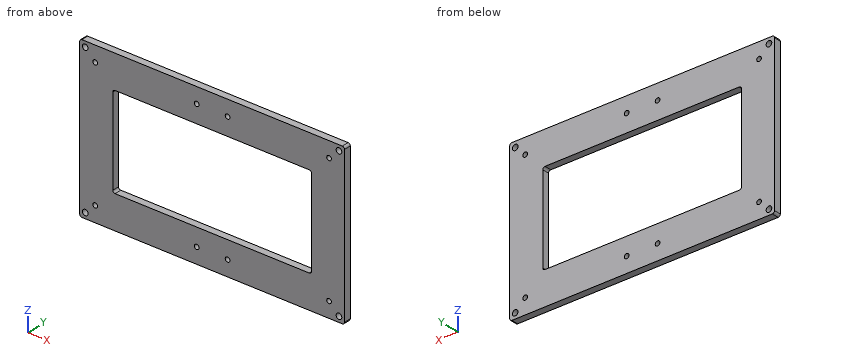
Autodesk Inventor part; units mm, degrees
ref_plane "YZ Plane" through (0, 0, 0) normal (1, 0, 0) x (0, 1, 0)
ref_plane "XZ Plane" through (0, 0, 0) normal (0, 1, 0) x (-1, 0, 0)
ref_plane "XY Plane" through (0, 0, 0) normal (0, 0, 1) x (1, 0, 0)
sketch "Sketch1" plane through (0, 0, 0) normal (0, 1, 0) x (-1, 0, 0)
  line L0 (-120, 71.5) -> (120, 71.5)
  line L1 (120, 71.5) -> (120, 41.5)
  line L2 (120, 41.5) -> (-120, 41.5)
  line L3 (-120, 41.5) -> (-120, 71.5)
  line L4 (-120, -41.5) -> (120, -41.5)
  line L5 (120, -41.5) -> (120, -71.5)
  line L6 (120, -71.5) -> (-120, -71.5)
  line L7 (-120, -71.5) -> (-120, -41.5)
  line L8 (168, 0) -> (-168, 0)
  line L9 (0, -100.1) -> (0, 100.1)
  line L10 (120, 41.5) -> (-120, 41.5)
  line L11 (-120, 41.5) -> (-120, -41.5)
  line L12 (-120, -41.5) -> (120, -41.5)
  line L13 (120, -41.5) -> (120, 41.5)
  line L14 (90, 41.5) -> (-90, 41.5)
  line L15 (-90, 41.5) -> (-90, -41.5)
  line L16 (-90, -41.5) -> (90, -41.5)
  line L17 (90, -41.5) -> (90, 41.5)
  line L18 (-115, 66.5) -> (115, 66.5) construction
  line L19 (115, 66.5) -> (115, -66.5) construction
  line L20 (115, -66.5) -> (-115, -66.5) construction
  line L21 (-115, -66.5) -> (-115, 66.5) construction
  point P0 (0, 0)
  point P1 (0, 41.5)
  dimension "d0" = 240
  dimension "d2" = 30
  dimension "d4" = 143
  dimension "d55" = 30
  dimension "d56" = 5
  dimension "d57" = 5
extrude "Extrusion1" add sketch "Sketch1" along normal blind 6.35 contours L0 L9 L2 L3 | L0 L1 L2 L9 | L2 L15 L8 L11 | L8 L15 L4 L11 | L13 L8 L17 L2 | L4 L9 L6 L7 | L13 L4 L17 L8 | L4 L5 L6 L9
sketch "Sketch2" plane through (0, 6.35, 0) normal (0, 1, 0) x (1, 0, 0)
  line L0 (-110, -61.5) -> (-10, -61.5)
  line L1 (-10, -61.5) -> (-10, 61.5)
  line L2 (-10, 61.5) -> (-110, 61.5)
  line L3 (-110, 61.5) -> (-110, -61.5)
  line L4 (-120, -71.5) -> (-120, 71.5)
  line L5 (-120, -71.5) -> (120, -71.5)
  line L6 (10, -61.5) -> (110, -61.5)
  line L7 (110, -61.5) -> (110, 61.5)
  line L8 (110, 61.5) -> (10, 61.5)
  line L9 (10, 61.5) -> (10, -61.5)
  circle A0 centre (-106, -57.5) radius 2.1
  circle A1 centre (-106, 57.5) radius 2.1
  circle A2 centre (-14, -57.5) radius 2.1
  circle A3 centre (-14, 57.5) radius 2.1
  circle A4 centre (14, -57.5) radius 2.1
  circle A5 centre (14, 57.5) radius 2.1
  circle A6 centre (106, -57.5) radius 2.1
  circle A7 centre (106, 57.5) radius 2.1
  point P0 (0, 0)
  point P1 (-120, -41.5)
  dimension "d7" = 123
  dimension "d8" = 100
  dimension "d9" = 10
  dimension "d10" = 10
  dimension "d11" = 100
  dimension "d12" = 123
  dimension "d13" = 20
  dimension "d14" = 4.2
  dimension "d15" = 4
  dimension "d16" = 4
  dimension "d17" = 4.2
  dimension "d18" = 4
  dimension "d19" = 4
  dimension "d20" = 4.2
  dimension "d21" = 4
  dimension "d22" = 4
  dimension "d23" = 4.2
  dimension "d24" = 4
  dimension "d25" = 4
  dimension "d26" = 4.2
  dimension "d27" = 4
  dimension "d28" = 4
  dimension "d29" = 4.2
  dimension "d30" = 4
  dimension "d31" = 4
  dimension "d32" = 4.2
  dimension "d33" = 4
  dimension "d34" = 4
  dimension "d35" = 4.2
  dimension "d36" = 4
  dimension "d37" = 4
  dimension "d38" = 10
extrude "Extrusion2" cut sketch "Sketch2" against normal through all contours A0 | A1 | A2 | A3 | A4 | A5 | A6 | A7
sketch "Sketch3" plane through (0, 6.35, 0) normal (0, 1, 0) x (1, 0, 0)
  circle A0 centre (-115, -66.5) radius 2.5
  line L0 (-120, -71.5) -> (-120, 71.5)
  line L1 (120, -71.5) -> (-120, -71.5)
  circle A1 centre (-115, 66.5) radius 2.5
  line L2 (-120, 41.5) -> (-120, 71.5)
  line L3 (-120, 71.5) -> (120, 71.5)
  circle A2 centre (115, -66.5) radius 2.5
  line L4 (120, -71.5) -> (120, 71.5)
  circle A3 centre (115, 66.5) radius 2.5
  line L5 (120, 41.5) -> (120, 71.5)
  point P0 (0, 0)
  point P1 (-120, -41.5)
  point P2 (120, -41.5)
  dimension "d41" = 5
  dimension "d42" = 5
  dimension "d43" = 5
  dimension "d44" = 5
  dimension "d45" = 5
  dimension "d46" = 5
  dimension "d47" = 5
  dimension "d48" = 5
  dimension "d49" = 5
  dimension "d50" = 5
  dimension "d51" = 5
  dimension "d52" = 5
extrude "Extrusion3" [suppressed]
hole "Hole1" at (115, 0, 66.5) at (115, 0, -66.5) at (-115, 0, -66.5) at (-115, 0, 66.5) direction (0, 1, 0) diameter 5.1 end through all
fillet "Fillet1" radius 2 8 edges at (90, 3.175, 41.5) (90, 3.175, -41.5) (-90, 3.175, 41.5) (-90, 3.175, -41.5) (-120, 3.175, 71.5) (-120, 3.175, -71.5) (120, 3.175, -71.5) (120, 3.175, 71.5)
sketch "Sketch5" plane through (0, 0, 0) normal (0, 1, 0) x (-1, 0, 0)
  point P0 (0, 0)
properties part number "BoardMountingBracket"
Verification items for the finished model (mm, model axes). Coordinates: 2 decimals unless noted, no trailing zeros. Write each loop counter-clockwise with the first axis right and the second up, starting at its lowest first coordinate (ties: lowest second). Pieces come first, ordered by that corner, then holes. Notation, with made-up numbers: M 64.25,35.5 L 105.25,35.5 A25 ccw 105.25,60.5 Z; hole C 42,-3.75 d9. An arc over 180 degrees is marked long. One line per question, with ' | ' between items.
1) Sectioned sample at B-B on y = 5.25. State how many separate pieces and enclosed holes the cut face has, then the cut area to 3 significant figures.
Solutions:
separate pieces: 1 | enclosed holes: 13 | area: 19,200 mm^2
2) Sectioned sample at C-C on x = 115. Record the cut outline in (y, z), then the cut area to 3 significant figures.
Solutions:
outline: M 0,-71.5 L 6.35,-71.5 L 6.35,-69.05 L 0,-69.05 Z; M 0,-63.95 L 6.35,-63.95 L 6.35,63.95 L 0,63.95 Z; M 0,69.05 L 6.35,69.05 L 6.35,71.5 L 0,71.5 Z | area: 843 mm^2
3) Depth check by flat-ended pin: pin 1 Ø4 at (x, z) = (14, 57.5) entering from +Y. Enter the tip coordinate at first touch or a pass-through.
Solutions:
pin 1: through
4) Sectioned sample at D-D on z = 9. Record the cut outline in (x, y).
Solutions:
outline: M -120,0 L -90,0 L -90,6.35 L -120,6.35 Z; M 90,0 L 120,0 L 120,6.35 L 90,6.35 Z
5) Sectioned sample at A-A on z = 66.5. Record the cut outline in (x, y).
Solutions:
outline: M -120,0 L -117.55,0 L -117.55,6.35 L -120,6.35 Z; M -112.45,0 L 112.45,0 L 112.45,6.35 L -112.45,6.35 Z; M 117.55,0 L 120,0 L 120,6.35 L 117.55,6.35 Z
6) Material ranges on L1, parallel to Z at x = -14, y = 2.25; L2, parallel to Z at x = -106, y = 4; L3, parallel to X at y = 2.25, z = -57.5, recorded low to high.
Solutions:
L1: -71.5 to -59.6, -55.4 to -41.5, 41.5 to 55.4, 59.6 to 71.5 | L2: -71.5 to -59.6, -55.4 to 55.4, 59.6 to 71.5 | L3: -120 to -108.1, -103.9 to -16.1, -11.9 to 11.9, 16.1 to 103.9, 108.1 to 120
